Drawing for the job (mm, zero at the part's lowest x, y, z). Round coordinates to 2 decimals unless told otherwise and drop trailing zeros. Write each loop counter-clockwise with the first axis right and the second up, starting at its lowest first coordinate (ties: lowest second). Pieces come first, ordered by that corner, then holes. Notation, with made-up numbers: (-32, -24) - (7, -24) arc R24 cw to (7, 8) - close; hole circle Ø1 at (73.5, -21). An arc over 180 degrees is marked (long way). Answer in a Markdown table with one row per item.
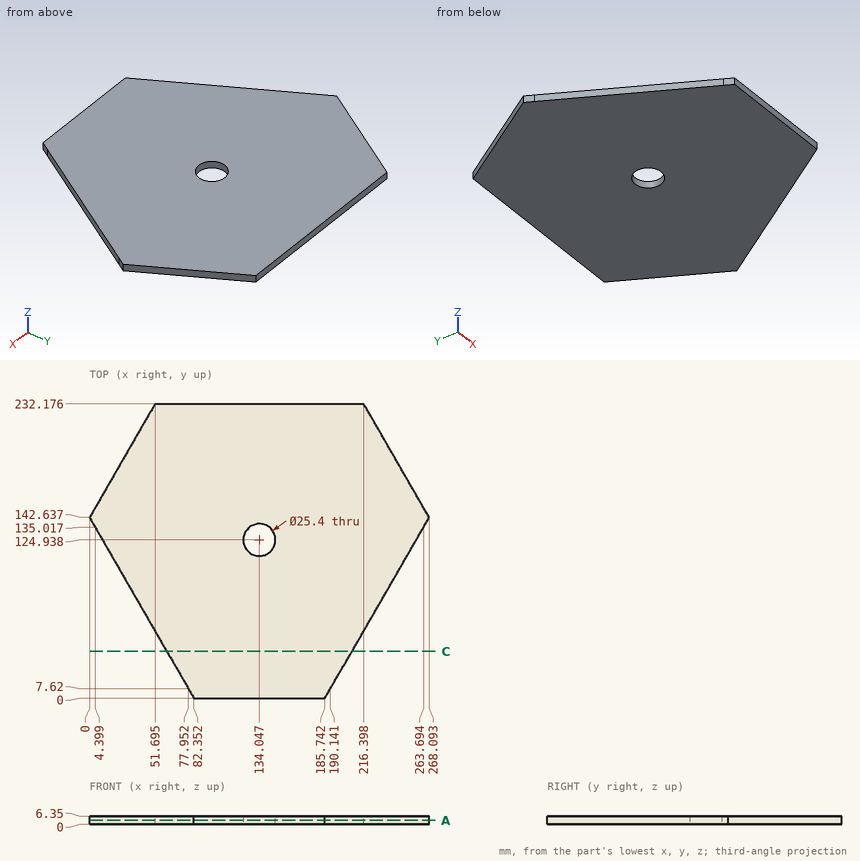
Q1. Saw through at C-C on y = 37. List the corners of the cut face in (x, z).
Computed:
| item | result |
|---|---|
| outline | (60.99, 0) - (207.1, 0) - (207.1, 6.35) - (60.99, 6.35) - close |
Q2. Flat gauge pins, fed straight in: pin 1 (3 mm diameter, centred on y = 90, z = 3, fed in from +X); pin 2 (15 mm diameter, centred on x = 134.05, y = 124.94, fed in from +Z). Where does each tip first touch, or does it go through?
Computed:
| item | result |
|---|---|
| pin 1 | stops at x = 238.57 |
| pin 2 | passes through |
Q3. Drill centre lines: line 1 (Y direction, x = 142.5, z = 0.5) (1 decimal); line 2 (Y direction, x = 138.5, z = 5.75) (1 decimal); line 3 (X direction, y = 114, z = 5) (1 decimal). Where is each one in solid material? Low to high.
Computed:
| item | result |
|---|---|
| line 1 | y = 0 to 115.5, 134.4 to 232.2 |
| line 2 | y = 0 to 113, 136.8 to 232.2 |
| line 3 | x = 16.5 to 127.6, 140.5 to 251.6 |
Q4. Saw through at A-A on z = 3. List the corners of the cut face in (x, y) (1 decimal), then the cut area to 3 significant figures.
Computed:
| item | result |
|---|---|
| outline | (0, 142.6) - (82.4, 0) - (185.7, 0) - (268.1, 142.6) - (216.4, 232.2) - (51.7, 232.2) - close; hole circle Ø25.4 at (134, 124.9) |
| area | 45,400 mm2 |
